```python
from build123d import *

# Parameters (mm, degrees)
SKETCH1_W                                     = 539
SKETCH1_H                                     = 299
BOSS_EXTRUDE1_DEPTH                           = 14.5
SKETCH22_W                                    = 70
SKETCH22_H                                    = 20
CUT_EXTRUDE9_DEPTH                            = 309.529982336
CUT_EXTRUDE1_DEPTH                            = 6
CSK_FOR_M4_COUNTERSUNK_FLAT_HEAD1_D           = 4.5
CSK_FOR_M4_COUNTERSUNK_FLAT_HEAD1_CSINK_D     = 9.4
CSK_FOR_M4_COUNTERSUNK_FLAT_HEAD1_CSINK_ANGLE = 90
MIRROR2_COPY_1_D                              = 4.5
MIRROR2_COPY_1_CSINK_D                        = 9.4
MIRROR2_COPY_1_CSINK_ANGLE                    = 90
SKETCH11_W                                    = 229
SKETCH11_H                                    = 168
CUT_EXTRUDE4_DEPTH                            = 2.245
SKETCH12_W                                    = 17
SKETCH12_H                                    = 168
BOSS_EXTRUDE2_DEPTH                           = 1.67
M6_CLEARANCE_HOLE1_D                          = 6.6
M4X0_7_TAPPED_HOLE1_D                         = 3.3
LPATTERN1_COUNT                               = 8
LPATTERN1_PITCH                               = 25
CUT_EXTRUDE5_DEPTH                            = 1.5
SKETCH21_W                                    = 20
SKETCH21_H                                    = 1.5
CUT_EXTRUDE8_DEPTH                            = 3.745


with BuildPart() as part:
    # Sketch1 → Boss-Extrude1 (new body)
    with BuildSketch(Plane(origin=(0, 0, 0), x_dir=(1, 0, 0), z_dir=(0, 1, 0))):
        Rectangle(SKETCH1_W, SKETCH1_H)
    extrude(amount=-BOSS_EXTRUDE1_DEPTH)

    # Sketch22 → Cut-Extrude9 (cut, through all)
    with BuildSketch(Plane(origin=(0, 0, 0), x_dir=(1, 0, 0), z_dir=(0, 1, 0))):
        Polygon((269.5, 149.5), (199.5, 149.5), (199.5, 129.5), (249.5, 129.5), (249.5, 91.5), (269.5, 91.5), align=None)
        with Locations((234.5, -139.5)):
            Rectangle(SKETCH22_W, SKETCH22_H)
    extrude(amount=-CUT_EXTRUDE9_DEPTH, mode=Mode.SUBTRACT)

    # Sketch2 → Cut-Extrude1 (cut)
    with BuildSketch(Plane.XZ.offset(14.5)):
        with BuildLine():
            Line((-234.5, -3), (-234.5, -89.5))
            Line((-234.5, -89.5), (-110.5, -89.5))
            Line((-110.5, -89.5), (-110.5, 93.5))
            Line((-110.5, 93.5), (-89, 93.5))
            Line((-89, 93.5), (-89, 128.5))
            Line((-89, 128.5), (178.5, 128.5))
            Line((178.5, 128.5), (178.5, 108.5))
            Line((178.5, 108.5), (228.5, 108.5))
            Line((228.5, 108.5), (228.5, -3))
            Line((228.5, -3), (260, -3))
            ThreePointArc((260, -3), (263, 0), (260, 3))
            Line((260, 3), (234.5, 3))
            Line((234.5, 3), (234.5, 114.5))
            Line((234.5, 114.5), (184.5, 114.5))
            Line((184.5, 114.5), (184.5, 134.5))
            Line((184.5, 134.5), (-95, 134.5))
            Line((-95, 134.5), (-95, 99.5))
            Line((-95, 99.5), (-130, 99.5))
            Line((-130, 99.5), (-130, -83.5))
            Line((-130, -83.5), (-228.5, -83.5))
            Line((-228.5, -83.5), (-228.5, 3))
            Line((-228.5, 3), (-260, 3))
            ThreePointArc((-260, 3), (-263, 0), (-260, -3))
            Line((-260, -3), (-234.5, -3))
        make_face()
    extrude(amount=-CUT_EXTRUDE1_DEPTH, mode=Mode.SUBTRACT)

    # CSK for M4 Countersunk Flat Head1 (through all)
    with Locations(Plane(origin=(-259.5, 0, -15), x_dir=(0, 0, 1), z_dir=(0, 1, 0))):
        with Locations((0, 0)):
            csk_for_m4_countersunk_flat_head1 = CounterSinkHole(CSK_FOR_M4_COUNTERSUNK_FLAT_HEAD1_D / 2, CSK_FOR_M4_COUNTERSUNK_FLAT_HEAD1_CSINK_D / 2, counter_sink_angle=CSK_FOR_M4_COUNTERSUNK_FLAT_HEAD1_CSINK_ANGLE)

    # Mirror1: CSK for M4 Countersunk Flat Head1 across plane
    add(csk_for_m4_countersunk_flat_head1.mirror(Plane.XY), mode=Mode.SUBTRACT)

    # Mirror2: CSK for M4 Countersunk Flat Head1 across plane
    add(csk_for_m4_countersunk_flat_head1.mirror(Plane(origin=(0, 0, 0), x_dir=(0, 0, 1), z_dir=(1, 0, 0))), mode=Mode.SUBTRACT)

    # Mirror2 copy 1 (through all)
    with Locations(Plane(origin=(259.5, 0, 15), x_dir=(0, 0, -1), z_dir=(0, 1, 0))):
        with Locations((0, 0)):
            CounterSinkHole(MIRROR2_COPY_1_D / 2, MIRROR2_COPY_1_CSINK_D / 2, counter_sink_angle=MIRROR2_COPY_1_CSINK_ANGLE)

    # Sketch11 → Cut-Extrude4 (cut)
    with BuildSketch(Plane.XZ.offset(14.5)):
        with Locations((14, 0)):
            Rectangle(SKETCH11_W, SKETCH11_H)
    extrude(amount=-CUT_EXTRUDE4_DEPTH, mode=Mode.SUBTRACT)

    # Sketch12 → Boss-Extrude2 (add)
    with BuildSketch(Plane.XZ.offset(12.255)):
        with Locations((-92, 0)):
            Rectangle(SKETCH12_W, SKETCH12_H)
    extrude(amount=BOSS_EXTRUDE2_DEPTH)

    # M6 Clearance Hole1 (through all)
    with Locations(Plane(origin=(-255, 0, -105), x_dir=(0, 0, 1), z_dir=(0, 1, 0))):
        with Locations((0, 0), (70, 0), (140, 0), (210, 0), (210, 85), (140, 85), (70, 85), (0, 85), (0, 170), (0, 255), (0, 340), (0, 425), (70, 510), (140, 510), (210, 510), (210, 425), (140, 425), (70, 425), (210, 340), (210, 255), (140, 255), (70, 255), (70, 340), (140, 340), (140, 170), (70, 170)):
            Hole(M6_CLEARANCE_HOLE1_D / 2)

    # M4x0.7 Tapped Hole1 (through all)
    with Locations(Plane(origin=(-120.25, -8.5, -81.5), x_dir=(0, 0, -1), z_dir=(0, -1, 0))):
        with Locations((0, 0)):
            m4x0_7_tapped_hole1 = Hole(M4X0_7_TAPPED_HOLE1_D / 2)

    # LPattern1: M4x0.7 Tapped Hole1 ×8
    with Locations(*[(0, 0, i * LPATTERN1_PITCH) for i in range(1, LPATTERN1_COUNT)]):
        add(m4x0_7_tapped_hole1, mode=Mode.SUBTRACT)

    # Sketch20 → Cut-Extrude5 (cut)
    with BuildSketch(Plane.XZ.offset(12.255)):
        Polygon((-63.5, -84), (-83.5, -84), (-83.5, -10), (-83.5, 10), (-83.5, 84), (-63.5, 84), (-63.5, 10), (-40.5, 10), (-40.5, 84), (-20.5, 84), (-20.5, 10), (12.5, 10), (12.5, 84), (32.5, 84), (32.5, 10), (65.5, 10), (65.5, 84), (85.5, 84), (85.5, 10), (108.5, 10), (108.5, 84), (128.5, 84), (128.5, -84), (108.5, -84), (108.5, -10), (85.5, -10), (85.5, -84), (65.5, -84), (65.5, -10), (32.5, -10), (32.5, -84), (12.5, -84), (12.5, -10), (-20.5, -10), (-20.5, -84), (-40.5, -84), (-40.5, -10), (-63.5, -10), align=None)
    extrude(amount=-CUT_EXTRUDE5_DEPTH, mode=Mode.SUBTRACT)

    # Sketch21 → Cut-Extrude8 (cut)
    with BuildSketch(Plane.XZ.offset(14.5)):
        with Locations((-73.5, -84.75)):
            Rectangle(SKETCH21_W, SKETCH21_H)
        with Locations((-30.5, -84.75)):
            Rectangle(SKETCH21_W, SKETCH21_H)
        with Locations((22.5, -84.75)):
            Rectangle(SKETCH21_W, SKETCH21_H)
        with Locations((75.5, -84.75)):
            Rectangle(SKETCH21_W, SKETCH21_H)
        with Locations((118.5, -84.75)):
            Rectangle(SKETCH21_W, SKETCH21_H)
    extrude(amount=-CUT_EXTRUDE8_DEPTH, mode=Mode.SUBTRACT)


solid = part.part
```
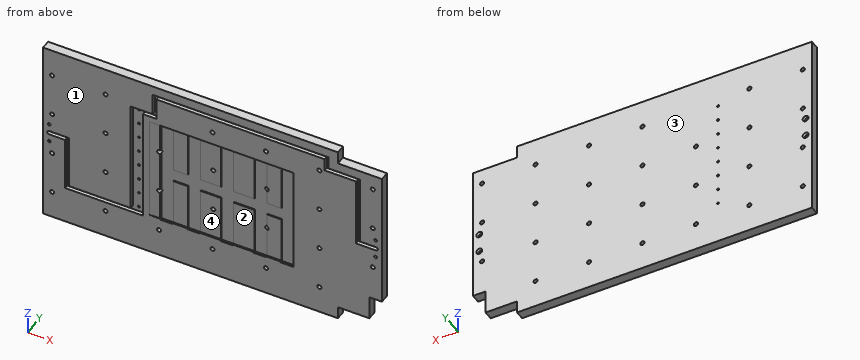
The model under review builds one solid part; all positions refer to its coordinate system, in mm. Face numbers are marked on the shaded views. A direction names the side the tool comes from. Give positions to 0.01 mm unless a question says otherwise; leave off trailing zeros. Write each loop counter-clockwise with the first axis right and the second up, starting at its lowest first coordinate (ties: lowest second). Pieces come first, ordered by that corner, then holes. Notation, with made-up numbers: (55.5, 45) - (92.5, 45) arc R26 ccw to (92.5, 83) - close; hole circle Ø8 at (-18.75, 33). An arc over 180 degrees is marked (long way). Answer in a Markdown table with one row per item. Add a question column.
1. We need section A-A on x = 100.5. Write out the cut boundary in (y, z) (3 decimals), then the cut area to 3 significant figures.
2. Wall thickness on line 1 along Z through (x, y) = (-255, -6); line 2 along Z through (x, y) = (19, -11); line 3 along X through (y, z) = (-6.75, -15): over which ranges is each line inside the solid? List them lowest first. Write a range as [from, to].
3. Insertion check: P1, Ø5.5, axis at x = -255, z = 105, coming from the +Y side. The pin has a flat end and moves straight along its axis. Give the tip position at first contact, or say it passes through.
4. Draft analysis for pull direction X (two halves, no side actions). For the marked faces 3 and 4, state which applies: +X half, -X half, draft (parallel to the pull), parting line (faces both ways), or undercut.
5. Tool access review of the marked faces 1 and 2: name each direction out of +Z, -Z, +X, -X, +Y, -Y from which nothing blocks a thin tool from reaching the whole face with its end or side.
Ans:
| question | item | result |
|---|---|---|
| 1 | outline | (-14.5, -149.5) - (0, -149.5) - (0, 149.5) - (-14.5, 149.5) - (-14.5, 134.5) - (-8.5, 134.5) - (-8.5, 128.5) - (-14.5, 128.5) - (-14.5, 84) - (-12.255, 84) - (-12.255, 10) - (-10.755, 10) - (-10.755, -10) - (-12.255, -10) - (-12.255, -84) - (-14.5, -84) - close |
| 1 | area | 3,890 mm^2 |
| 2 | line 1 | z = [-149.5, -108.3], [-101.7, -38.3], [-31.7, 31.7], [38.3, 101.7], [108.3, 149.5] |
| 2 | line 2 | z = [-149.5, -85.5], [84, 128.5], [134.5, 149.5] |
| 2 | line 3 | x = [-269.5, -261.75], [-257.25, 257.25], [261.75, 269.5] |
| 3 | P1 | passes through |
| 4 | face 3 | draft |
| 4 | face 4 | undercut |
| 5 | face 1 | +Z, -Z, +X, -X, -Y |
| 5 | face 2 | -Y |
